CAD build for the part. Positions are in the model's coordinates, mm. A direction names the side the tool comes from. Give positions to 0.01 mm unless a question says otherwise; leave off trailing zeros. Write each loop counter-clockwise with the first axis right and the second up, starting at its lowest first coordinate (ties: lowest second). Pieces come first, ordered by that corner, then holes. Notation, with made-up numbers: (87, 12.5) - (92, 12.5) arc R14 ccw to (92, 35.5) - close; hole circle Ø5 at (18.5, 8). An arc over 180 degrees is marked (long way). Put each result on its own line as item: value. Start each with the question number.
1. Cut at D-D on x = -15. List the corners of the cut face in (y, z).
2. Wall check: line 1 (Y direction, x = 10, z = -1); line 2 (Z direction, x = 15.5, y = -8.5); line 3 (Y direction, x = 11, z = -1). Give the ranges that are in metal, low to high.
3. Cut at A-A on y = 0. List the corners of the cut face in (x, z), and give its area (3 significant figures).
4. Cut at C-C on z = -7. List the corners of the cut face in (x, y).
5. Tool access for faces 1 (the flat face through (0, 21.15, -52)), 2 (the cylindrical face through (9.574, -11.364, -2.465)): list every direction of +Z, -Z, +X, -X, +Y, -Y with a clear straight run to the whole face (end or side of a thin tool).
6. Mould opens along X. For faces 3 (the flat face through (10, 10, -5)), 4 (the flat face through (10, -10, -5)), 5 (the cylindrical face through (-3, 0, 10)), 6 (the flat face through (-21.15, 0, -52)) say: +X half, -X half, draft (parallel to the pull), parting line (faces both ways), or undercut.
7. Drop flat-ended pins along their axis: pin 1 (4 mm diameter, centred on x = -14.5, y = -7, fed in from +Z); pin 2 (2.5 mm diameter, centred on x = 9.9, y = 9.9, fed in from +Z); pin 3 (3 mm diameter, centred on y = -1.5, z = -22, fed in from -X); pin 4 (5 mm diameter, centred on y = -9, z = 6.5, fed in from +X). Give the stop position or say it passes through.
from build123d import *

# Parameters (mm, degrees)
SKETCH_R     = 18
PAD_DEPTH    = 35
SKETCH001_W  = 42.3
SKETCH001_H  = 42.3
PAD001_DEPTH = 34
SKETCH002_R  = 11
PAD002_DEPTH = 2
SKETCH003_R  = 3
PAD003_DEPTH = 18
SKETCH004_R  = 1.5
POCKET_DEPTH = 5


with BuildPart() as part:
    # Sketch → Pad (new body)
    with BuildSketch(Plane.XY):
        Circle(SKETCH_R)
    extrude(amount=-PAD_DEPTH)

    # Sketch001 → Pad001 (join)
    with BuildSketch(Plane.XY.offset(-35)):
        Rectangle(SKETCH001_W, SKETCH001_H)
    extrude(amount=-PAD001_DEPTH)

    # Sketch002 → Pad002 (join)
    with BuildSketch(Plane.XY):
        Circle(SKETCH002_R)
    extrude(amount=PAD002_DEPTH)

    # Sketch003 → Pad003 (join)
    with BuildSketch(Plane.XY):
        Circle(SKETCH003_R)
    extrude(amount=PAD003_DEPTH)

    # Sketch004 → Pocket (cut)
    with BuildSketch(Plane.XY):
        with Locations((-9.899495, 9.899495)):
            Circle(SKETCH004_R)
        with Locations((9.899495, 9.899495)):
            Circle(SKETCH004_R)
        with Locations((9.899495, -9.899495)):
            Circle(SKETCH004_R)
        with Locations((-9.899495, -9.899495)):
            Circle(SKETCH004_R)
    extrude(amount=-POCKET_DEPTH, mode=Mode.SUBTRACT)


solid = part.part
Report:
1. outline: (-21.15, -69) - (21.15, -69) - (21.15, -35) - (9.95, -35) - (9.95, 0) - (-9.95, 0) - (-9.95, -35) - (-21.15, -35) - close
2. line 1: y = -14.97 to -11.4, -8.4 to 8.4, 11.4 to 14.97
2. line 2: z = -69 to 0
2. line 3: y = -14.25 to -10.92, -8.88 to 8.88, 10.92 to 14.25
3. outline: (-21.15, -69) - (21.15, -69) - (21.15, -35) - (18, -35) - (18, 0) - (11, 0) - (11, 2) - (3, 2) - (3, 18) - (-3, 18) - (-3, 2) - (-11, 2) - (-11, 0) - (-18, 0) - (-18, -35) - (-21.15, -35) - close
3. area: 2,840 mm²
4. outline: circle Ø36 at (0, 0)
5. face 1: +Z, -Z, +X, -X, +Y
5. face 2: +Z
6. face 3: undercut
6. face 4: undercut
6. face 5: parting line
6. face 6: -X half
7. pin 1: stops at z = 0
7. pin 2: stops at z = -5
7. pin 3: stops at x = -18
7. pin 4: passes through
